```python
from build123d import *

# Parameters (mm, degrees)
F0_R         = 39
F0_R_2       = 38.1
F1_DEPTH     = 9
F2_DEPTH     = 10
F0_W         = 32
F0_H         = 32
F3_DEPTH     = 2.5
F5_R         = 38.8254389769
F6_DEPTH     = 2
F7_R         = 0.99999
F9_DEPTH     = 12.5
F10_DEPTH    = 12.5
F11_DEPTH    = 2.5
F12_T2_ANGLE = 166.0974661722
F13_DEPTH    = 14
F14_R        = 0.5


# Not quite as in the source:
# - a fillet or chamfer that OpenCascade refuses, or shapes differently, is made with other operations: its cross-section is extruded or revolved along the edge and cut away or added
# - a fillet or chamfer is up to 0.001 mm smaller than in the source, because OpenCascade refuses the exact size


with BuildPart() as f1:
    # F0 (on Top) → F1 (new body)
    with BuildSketch(Plane.XY):
        Circle(F0_R)
        Circle(F0_R_2, mode=Mode.SUBTRACT)
    extrude(amount=F1_DEPTH)

    # F0 (on Top) → F2 (join)
    with BuildSketch(Plane.XY):
        Circle(F0_R)
        Circle(F0_R_2, mode=Mode.SUBTRACT)
    extrude(amount=F2_DEPTH)

    # F5 (on offset) → F6 (join)
    with BuildSketch(Plane.XY.offset(9)):
        Circle(F5_R)
    extrude(amount=F6_DEPTH)

    # F7 (radius 1 in the source; OpenCascade refuses exactly that, so slightly less here)
    f7_edges = [f1.edges().sort_by_distance(p)[0] for p in [
        (-38.825439, 0, 11),
    ]]
    fillet(f7_edges, radius=F7_R)


with BuildPart() as f3:
    # F0 (on Top) → F3 (new body)
    with BuildSketch(Plane.XY):
        Circle(F0_R_2)
        Rectangle(F0_W, F0_H, mode=Mode.SUBTRACT)
    extrude(amount=-F3_DEPTH)


with BuildPart() as f9:
    # F8 (on Top) → F9 (new body, symmetric)
    with BuildSketch(Plane.XY):
        Polygon((-41.2051826715, 48.0051673949), (-42.0097357945, 0), (0, 0), (36.1852608621, -14.1163477674), (49.7808791697, -14.1163477674), (49.2908842862, 48.0051673949), align=None)
    extrude(amount=F9_DEPTH, both=True)


with BuildPart() as f10_tool:
    # F8 (on Top) → F10 (new body, symmetric)
    with BuildSketch(Plane.XY):
        Polygon((-41.2051826715, 48.0051673949), (-42.0097357945, 0), (0, 0), (36.1852608621, -14.1163477674), (49.7808791697, -14.1163477674), (49.2908842862, 48.0051673949), align=None)
    extrude(amount=F10_DEPTH, both=True)


with BuildPart() as f1_1:
    add(f1.part)

    # F10: cut by f10_tool
    add(f10_tool.part, mode=Mode.SUBTRACT)


with BuildPart() as f3_1:
    add(f3.part)

    # F10: cut by f10_tool
    add(f10_tool.part, mode=Mode.SUBTRACT)


with BuildPart() as f9_1:
    add(f9.part)

    # F10: cut by f10_tool
    add(f10_tool.part, mode=Mode.SUBTRACT)


with BuildPart() as f11:
    # F11 (new): a face of the model
    f11_faces = [f1_1.part.faces().sort_by_distance(p)[0] for p in [
        (-38.55, -0.8484965841, 0),
    ]]
    extrude(f11_faces, amount=F11_DEPTH)

    # F12: fillet of radius 1 on 1 edges, made by hand

    # F12_s1 → F12_t2 (revolve, cut)
    with BuildSketch(Plane(origin=(0, 0, 0), x_dir=(0, 0, 1), z_dir=(0.0638176413, 0.9979615767, 0))):
        with BuildLine():
            ThreePointArc((-1.5050125629, -39), (-2.1758329561, -38.7416198487), (-2.5, -38.1))
            Line((-2.5, -38.1), (-2.5, -39))
            Line((-2.5, -39), (-1.5050125629, -39))
        make_face()
    revolve(axis=Axis((0, 0, -2.5), (0, 0, 1)), revolution_arc=F12_T2_ANGLE, mode=Mode.SUBTRACT)


with BuildPart() as f1_2:
    add(f1_1.part)

    # F13 (add): a face of the model
    f13_faces = [f3_1.part.faces().sort_by_distance(p)[0] for p in [
        (-27.05, 0, -1.25),
    ]]

    add(f3_1.part)  # F13 merges F3

    add(f11.part)  # F13 merges F11
    extrude(f13_faces, amount=F13_DEPTH)

    # F14
    f14_edges = [f1_2.edges().sort_by_distance(p)[0] for p in [
        (-27.05, 14, -2.5),
        (-27.05, 14, 0),
    ]]
    fillet(f14_edges, radius=F14_R)


solid = f1_2.part
```
Part model, mm, in its own coordinate system. A direction names the side the tool comes from. Round coordinates to 2 decimals unless told otherwise and drop trailing zeros. Loops run counter-clockwise (first coordinate to the right, second up) from the corner with the lowest first, then second, coordinate; pieces in that order, holes last. Notation, with made-up numbers: (-12.5, 60) -> (-8.5, 60) arc R35 cw to (-8.5, 95) -> close; hole circle Ø10 at (-19, 16). An arc over 180 degrees is marked (long way). Use one line per item in the form item = value. Start each with the question number.
Item 1: Drop flat-ended pins along their axis: pin 1 Ø0.8 at (y, z) = (-11, -1) entering from -X; pin 2 Ø1.2 at (x, z) = (1, -1) entering from +Y; pin 3 Ø2 at (y, z) = (-19, 3) entering from -X; pin 4 Ø1.5 at (y, z) = (2.5, 5) entering from -X. Give the stop position or say it passes through.
Item 2: Band-saw the part on B-B (z = 4.5). List the corners of the cut face in (x, y).
Item 3: Two-plate mould, pull along Z, no slides. Class faces 1 (the flat face through (-10, -18, 0)), 2 (the flat face through (-16, -1, -1)), 3 (the flat face through (-10, -18, -2.5)), 4 (the cylindrical face through (-7.77, -37.3, 4.44)): released by +Z, released by -Z, zero draft, split by the parting line, or undercut.
Item 4: Tool access for faces 5 (the flat face through (-38.1, 7, -1)), 6 (the flat face through (-2, -19, 9)), 7 (the flat face through (16, -11, -1)): list every direction of +Z, -Z, +X, -X, +Y, -Y with a clear straight run to the whole face (end or side of a thin tool).
Item 5: Drill centre lines: line 1 along Z through (x, y) = (1, -33); line 2 along Z through (x, y) = (-6, -11.5); line 3 along X through (y, z) = (-32, 2.25). Where is each one in solid material? Low to high.
Item 6: Band-saw the part on A-A (y = 8). List the corners of the cut face in (x, z), plus the area to 4 significant figures.
Data:
q1.pin_1 = -37.53
q1.pin_2 = -16
q1.pin_3 = -34.6
q1.pin_4 = through
q2.outline = (-39, 0) arc R39 ccw to (36.36, -14.12) -> (36.19, -14.12) -> (35.49, -13.85) arc R38.1 cw to (-38.1, 0) -> close
q3.face_1 = undercut
q3.face_2 = zero draft
q3.face_3 = released by -Z
q3.face_4 = undercut
q4.face_5 = +Z, -Z, -X, +Y
q4.face_6 = +Y
q4.face_7 = -Z, +Y
q5.line_1 = -2.5 to 0, 9 to 11
q5.line_2 = 9 to 11
q5.line_3 = -22.29 to -20.68, 20.68 to 22.29
q6.outline = (-38.1, -2.5) -> (-16, -2.5) -> (-16, 0) -> (-38.1, 0) -> close
q6.area = 55.25 mm^2
